```python
from build123d import *

# Parameters (mm, degrees)
SKETCH1_R           = 1.5
SKETCH1_R_2         = 11
BOSS_EXTRUDE1_DEPTH = 6


with BuildPart() as part:
    # Sketch1 → Boss-Extrude1 (new body)
    with BuildSketch(Plane.XY):
        with BuildLine():
            Line((24.453034096, 353.905456547), (33.903511888, 338.683406525))
            ThreePointArc((33.903511888, 338.683406525), (36.546364709, 336.204527868), (40.074581718, 335.379182388))
            Line((40.074581718, 335.379182388), (57.982502631, 335.952511222))
            ThreePointArc((57.982502631, 335.952511222), (61.450700931, 337.001849574), (63.929579589, 339.644702395))
            Line((63.929579589, 339.644702395), (72.38702271, 355.440081251))
            ThreePointArc((72.38702271, 355.440081251), (73.21236819, 358.968298261), (72.163029838, 362.436496561))
            Line((72.163029838, 362.436496561), (62.712552046, 377.658546583))
            ThreePointArc((62.712552046, 377.658546583), (60.069699226, 380.137425241), (56.541482216, 380.962770721))
            Line((56.541482216, 380.962770721), (38.633561304, 380.389441887))
            ThreePointArc((38.633561304, 380.389441887), (35.165363003, 379.340103535), (32.686484345, 376.697250714))
            Line((32.686484345, 376.697250714), (24.229041225, 360.901871858))
            ThreePointArc((24.229041225, 360.901871858), (23.403695744, 357.373654848), (24.453034096, 353.905456547))
        make_face()
        with Locations((57.758509759, 342.948926532)):
            Circle(SKETCH1_R, mode=Mode.SUBTRACT)
        with Locations((48.308031967, 358.170976554)):
            Circle(SKETCH1_R_2, mode=Mode.SUBTRACT)
        with Locations((56.765475088, 373.966355411)):
            Circle(SKETCH1_R, mode=Mode.SUBTRACT)
        with Locations((30.400111055, 357.59764772)):
            Circle(SKETCH1_R, mode=Mode.SUBTRACT)
    extrude(amount=BOSS_EXTRUDE1_DEPTH)


solid = part.part
```
Check sheet for the modelled part. Datum: model origin and axes. Units: mm. Coordinates: 2 decimals unless noted, no trailing zeros. Write each loop counter-clockwise with the first axis right and the second up, starting at its lowest first coordinate (ties: lowest second). Pieces come first, ordered by that corner, then holes. Notation, with made-up numbers: (55, -3.5) -> (63, -3.5) arc R20 cw to (63, 9.5) -> close; hole circle Ø5 at (-1, -29). An arc over 180 degrees is marked (long way). Use a Markdown table: item, result.
1. Scan lines: line 1 along X through (y, z) = (357, 3.3); line 2 along X through (y, z) = (355.5, 2.05); line 3 along X through (y, z) = (356, 4.75). Record each from-to range of solid material in increasing order.
Reported:
| item | result |
|---|---|
| line 1 | x = 23.43 to 29.02, 31.78 to 37.37, 59.25 to 73 |
| line 2 | x = 23.72 to 37.64, 58.98 to 72.42 |
| line 3 | x = 23.58 to 37.52, 59.09 to 72.66 |
2. Go/stop test with flat-tipped pins: pin 1 Ø2 at (y, z) = (374.5, 1.5) entering from -X; pin 2 Ø2 at (y, z) = (372.5, 2) entering from +X; pin 3 Ø1 at (y, z) = (343.5, 2) entering from -X. Record where each tip stops, or that it passes through.
Reported:
| item | result |
|---|---|
| pin 1 | stops at x = 30.97 |
| pin 2 | stops at x = 66.54 |
| pin 3 | stops at x = 30.6 |
3. Sectioned sample at B-B (x = 53). Enter the section's corners in (y, z), plus the area to 3 significant figures.
Reported:
| item | result |
|---|---|
| outline | (335.79, 0) -> (348.22, 0) -> (348.22, 6) -> (335.79, 6) -> close; (368.12, 0) -> (380.85, 0) -> (380.85, 6) -> (368.12, 6) -> close |
| area | 151 mm2 |
4. Sectioned sample at D-D (z = 3.85). Enter the section's corners in (x, y).
Reported:
| item | result |
|---|---|
| outline | (24.23, 360.9) arc R7 ccw to (24.45, 353.91) -> (33.9, 338.68) arc R7 ccw to (40.07, 335.38) -> (57.98, 335.95) arc R7 ccw to (63.93, 339.64) -> (72.39, 355.44) arc R7 ccw to (72.16, 362.44) -> (62.71, 377.66) arc R7 ccw to (56.54, 380.96) -> (38.63, 380.39) arc R7 ccw to (32.69, 376.7) -> close; hole circle Ø3 at (30.4, 357.6); hole circle Ø22 at (48.31, 358.17); hole circle Ø3 at (56.77, 373.97); hole circle Ø3 at (57.76, 342.95) |
5. Sectioned sample at C-C (y = 357). Enter the section's corners in (x, z).
Reported:
| item | result |
|---|---|
| outline | (23.43, 0) -> (29.02, 0) -> (29.02, 6) -> (23.43, 6) -> close; (31.78, 0) -> (37.37, 0) -> (37.37, 6) -> (31.78, 6) -> close; (59.25, 0) -> (73, 0) -> (73, 6) -> (59.25, 6) -> close |
6. Sectioned sample at A-A (y = 363.5). Enter the section's corners in (x, z).
Reported:
| item | result |
|---|---|
| outline | (25.62, 0) -> (38.69, 0) -> (38.69, 6) -> (25.62, 6) -> close; (57.93, 0) -> (71.5, 0) -> (71.5, 6) -> (57.93, 6) -> close |
7. Release check for a two-part mould opening along X. For faces 1 (the flat face through (37, 358, 6)), 2 (the cylindrical face through (45.923, 347.433, 2.958)), 3 (the flat face through (67.504, 369.941, 2.958)), 4 (the cylindrical face through (23.402, 357.425, 2.958)) record: pulls with the +X half, pulls with the -X half, needs draft (parallel to the pull), parting line crosses it, or undercut.
Reported:
| item | result |
|---|---|
| face 1 | needs draft |
| face 2 | undercut |
| face 3 | pulls with the +X half |
| face 4 | pulls with the -X half |
